```python
from build123d import *

# Parameters (mm, degrees)
SKETCH1_W            = 140
SKETCH1_H            = 100
BOSS_EXTRUDE1_DEPTH  = 10
SKETCH2_W            = 10
SKETCH2_H            = 100
BOSS_EXTRUDE2_DEPTH  = 120
BOSS_EXTRUDE3_DEPTH  = 10
BOSS_EXTRUDE4_DEPTH  = 10
BOSS_EXTRUDE6_DEPTH  = 140
SKETCH7_W            = 120
SKETCH7_H            = 98.500973615
CUT_EXTRUDE1_DEPTH   = 30
SKETCH8_R            = 15
CUT_EXTRUDE2_DEPTH   = 170
SKETCH9_R            = 15
CUT_EXTRUDE3_DEPTH   = 170
CUT_EXTRUDE4_DEPTH   = 140
SKETCH14_W           = 120
SKETCH14_H           = 70
CUT_EXTRUDE5_DEPTH   = 10
BOSS_EXTRUDE8_DEPTH  = 10
BOSS_EXTRUDE9_DEPTH  = 10
SKETCH17_R           = 7.5
BOSS_EXTRUDE10_DEPTH = 120


with BuildPart() as part:
    # Sketch1 → Boss-Extrude1 (new body)
    with BuildSketch(Plane.XY):
        Rectangle(SKETCH1_W, SKETCH1_H)
    extrude(amount=BOSS_EXTRUDE1_DEPTH)

    # Sketch2 → Boss-Extrude2 (add)
    with BuildSketch(Plane.XY.offset(10)):
        with Locations((65, 0)):
            Rectangle(SKETCH2_W, SKETCH2_H)
        with Locations((-65, 0)):
            Rectangle(SKETCH2_W, SKETCH2_H)
    extrude(amount=BOSS_EXTRUDE2_DEPTH)

    # Sketch3 → Boss-Extrude3 (add)
    with BuildSketch(Plane.ZY.offset(70)):
        Polygon((130, 50), (145, 50), (135, -50), (130, -50), align=None)
    extrude(amount=-BOSS_EXTRUDE3_DEPTH)

    # Sketch4 → Boss-Extrude4 (add)
    with BuildSketch(Plane(origin=(70, 0, 0), x_dir=(0, 0, -1), z_dir=(1, 0, 0))):
        Polygon((-130, 50), (-145, 50), (-135, -50), (-130, -50), align=None)
    extrude(amount=-BOSS_EXTRUDE4_DEPTH)

    # Sketch6 → Boss-Extrude6 (add)
    with BuildSketch(Plane.ZY.offset(70)):
        Polygon((72.5, 90), (145, 170), (145, 50), (72.5, 50), (36.751913988, 50), align=None)
    extrude(amount=-BOSS_EXTRUDE6_DEPTH)

    # Sketch7 → Cut-Extrude1 (cut)
    with BuildSketch(Plane.XZ.offset(-50)):
        with Locations((0, 95.749513193)):
            Rectangle(SKETCH7_W, SKETCH7_H)
    extrude(amount=-CUT_EXTRUDE1_DEPTH, mode=Mode.SUBTRACT)

    # Sketch8 → Cut-Extrude2 (cut)
    with BuildSketch(Plane.ZY.offset(70)):
        with Locations((62.387439839, 0)):
            Circle(SKETCH8_R)
    extrude(amount=-CUT_EXTRUDE2_DEPTH, mode=Mode.SUBTRACT)

    # Sketch9 → Cut-Extrude3 (cut)
    with BuildSketch(Plane.XY.offset(10)):
        Circle(SKETCH9_R)
    extrude(amount=-CUT_EXTRUDE3_DEPTH, mode=Mode.SUBTRACT)

    # Sketch13 → Cut-Extrude4 (cut)
    with BuildSketch(Plane.ZY.offset(70)):
        Polygon((70.157530745, 70), (136.03947853, 146.817766748), (136.03947853, 70), align=None)
    extrude(amount=-CUT_EXTRUDE4_DEPTH, mode=Mode.SUBTRACT)

    # Sketch14 → Cut-Extrude5 (cut)
    with BuildSketch(Plane.XY.offset(145)):
        with Locations((0, 115)):
            Rectangle(SKETCH14_W, SKETCH14_H)
    extrude(amount=-CUT_EXTRUDE5_DEPTH, mode=Mode.SUBTRACT)

    # Sketch15 → Boss-Extrude8 (add)
    with BuildSketch(Plane.ZY.offset(70)):
        Polygon((136.03947853, 146.817766748), (136.03947853, 70), (70.157530745, 70), align=None)
    extrude(amount=-BOSS_EXTRUDE8_DEPTH)

    # Sketch16 → Boss-Extrude9 (add)
    with BuildSketch(Plane(origin=(70, 0, 0), x_dir=(0, 0, -1), z_dir=(1, 0, 0))):
        Polygon((-136.03947853, 146.817766748), (-136.03947853, 70), (-70.157530745, 70), align=None)
    extrude(amount=-BOSS_EXTRUDE9_DEPTH)

    # Sketch17 → Boss-Extrude10 (add)
    with BuildSketch(Plane.ZY.offset(-60)):
        with Locations((122.863088973, 101.43242494)):
            Circle(SKETCH17_R)
    extrude(amount=BOSS_EXTRUDE10_DEPTH)


solid = part.part
```
Check sheet for the modelled part. Datum: model origin and axes. Units: mm. A direction names the side the tool comes from. Give positions to 0.01 mm unless a question says otherwise; leave off trailing zeros. Write each loop counter-clockwise with the first axis right and the second up, starting at its lowest first coordinate (ties: lowest second). Pieces come first, ordered by that corner, then holes. Notation, with made-up numbers: (-7.75, 89.25) - (1.25, 89.25) arc R22 ccw to (1.25, 98.25) - close; hole circle Ø7 at (17.25, -11). An arc over 180 degrees is marked (long way). Answer as a JSON object with one key per item and string values. Group by question number.
1) Sectioned sample at D-D (x = -57.5). Record the cut outline in (y, z).
2) Sectioned sample at A-A (y = 0). Record the cut outline in (x, z), then the cut area to 3 significant figures.
3) Thickness scan on probe 1 along Y at (x, z) = (0, 7.25); probe 2 along X at (y, z) = (1, 35); probe 3 along Z at (x, y) = (-34.5, 0.5). Record the ranges inside material, lowest first. Write a range as from..to.
4) Sectioned sample at B-B (x = 11.5). Record the cut outline in (y, z).
5) Sectioned sample at C-C (z = 53). Record the cut outline in (x, y).
6) Access from +Z, -Z, +X, -X, +Y, -Y to the whole of each face (thin tool, end or side, straight path). Record for faces 5 (the face through (-0.84, 112.34, 106.47)), 6 (the face through (64.93, 0.66, 47.4)), 7 (the face through (-14, 12, 10)), 8 (the face through (1, 50, 6)), 9 (the face through (-1, 50, 42)).
7) Depth check by flat-ended pin: P1, Ø4.5, axis at x = -14.5, z = 69.5, coming from the -Y side; P2, Ø10, axis at x = 35, y = 31, coming from the +Z side; P3, Ø5.5, axis at x = 10, y = 54.5, coming from the +Z side. Enter the tip coordinate at first touch or a pass-through.
8) Release check for a two-part mould opening along Y. For faces 1 (the face through (-1, 150, 140)), 2 (the face through (0.84, 108.87, 121.89)), 3 (the face through (-0.98, 129.44, 108.24)), 4 (the face through (70, 37, 90)) record: pulls with the +Y half, pulls with the -Y half, needs draft (parallel to the pull), parting line crosses it, or undercut.
Geometry results:
{
 "1": {"outline": "(-50, 0) - (50, 0) - (50, 10) - (-50, 10) - close; (50, 36.75) - (60.91, 46.5) - (50, 46.5) - close; (80, 63.56) - (90, 72.5) - (170, 145) - (150, 145) - (150, 135) - (145.61, 135) - (80, 78.73) - close; circle Ø15 at (101.43, 122.86)"},
 "2": {"outline": "(-70, 0) - (-15, 0) - (-15, 10) - (-60, 10) - (-60, 47.39) - (-70, 47.39) - close; (-70, 77.39) - (-60, 77.39) - (-60, 140) - (-70, 140) - close; (15, 0) - (70, 0) - (70, 47.39) - (60, 47.39) - (60, 10) - (15, 10) - close; (60, 77.39) - (70, 77.39) - (70, 140) - (60, 140) - close", "area": "3,100 mm^2"},
 "3": {"probe 1": "y = -50..-15, 15..50", "probe 2": "x = -70..-60, 60..70", "probe 3": "z = 0..10"},
 "4": {"outline": "(-50, 0) - (-9.63, 0) - (-9.63, 10) - (-50, 10) - close; (9.63, 0) - (50, 0) - (50, 10) - (9.63, 10) - close; (50, 36.75) - (60.91, 46.5) - (50, 46.5) - close; (80, 63.56) - (90, 72.5) - (170, 145) - (150, 145) - (150, 135) - (145.61, 135) - (80, 78.73) - close; circle Ø15 at (101.43, 122.86)"},
 "5": {"outline": "(-70, -50) - (-60, -50) - (-60, -11.7) - (-70, -11.7) - close; (-70, 11.7) - (-60, 11.7) - (-60, 68.18) - (-70, 68.18) - close; (60, -50) - (70, -50) - (70, -11.7) - (60, -11.7) - close; (60, 11.7) - (70, 11.7) - (70, 68.18) - (60, 68.18) - close"},
 "6": {"face 5": "none", "face 6": "+X, -X", "face 7": "+Z, +Y, -Y", "face 8": "-Z, +X, -X, +Y", "face 9": "+Z, -Y"},
 "7": {"P1": "stops at y = 80", "P2": "stops at z = 10", "P3": "stops at z = 46.5"},
 "8": {"face 1": "pulls with the -Y half", "face 2": "undercut", "face 3": "pulls with the +Y half", "face 4": "needs draft"}
}
